The listing builds one solid part. Answer for the finished solid, in the listing's coordinates (mm). A direction names the side the tool comes from. Round coordinates to 2 decimals unless told otherwise and drop trailing zeros. Write each loop counter-clockwise with the first axis right and the second up, starting at its lowest first coordinate (ties: lowest second). Pieces come first, ordered by that corner, then holes.
(1) A cutting plane is placed at D-D, the plane y = 15. Give the vertices of the cut face in (x, z), and give its area (3 significant figures).
(2) Each of these flat-tipped pins is pushed along its axis until it touches: pin 1 Ø4 at (x, y) = (7, 7) entering from +Z; pin 2 Ø2 at (x, z) = (-1, 1) entering from -Y; pin 3 Ø2 at (y, z) = (11, 0) entering from +X. Where does it stop, or does it pass through?
(3) For faces 1 (the face through (-1, 1, 8)), 2 (the face through (-2.579, 4.93, -1.978)), 3 (the face through (-5, 0.49, -7.84)), determine the directions among +Z, -Z, +X, -X, +Y, -Y from which every point of the face is accessible in a straight line to the end or side of a thin tool.
(4) A cutting plane is placed at C-C, the plane z = 0. Give the vertices of the cut face in (x, y).
(5) Find the intervals of material crossed by probe 1 along Z at (x, y) = (0, 6.5); probe 2 along Y at (x, z) = (-2.75, -0.5); probe 3 along Y at (x, z) = (4.25, 6.5), in increasing order.
(6) The mould has two halves that part along Z. Classify faces 4 (the face through (0, 10, 0)), 5 (the face through (-4, 0, 0)), 6 (the face through (-7.493, 9.628, 0.33)): +Z half, -Z half, draft (parallel to the pull), parting line (faces both ways), or undercut.
(7) A cutting plane is placed at B-B, the plane x = 0. Give the vertices of the cut face in (y, z), and give its area (3 significant figures).
(8) A cutting plane is placed at A-A, the plane y = 8.25. Give the vertices of the cut face in (x, z).
Autodesk Inventor part; units mm, degrees
ref_plane "YZ Plane" through (0, 0, 0) normal (1, 0, 0) x (0, 1, 0)
ref_plane "XZ Plane" through (0, 0, 0) normal (0, 1, 0) x (-1, 0, 0)
ref_plane "XY Plane" through (0, 0, 0) normal (0, 0, 1) x (1, 0, 0)
sketch "Esboço1" plane through (0, 0, 0) normal (0, 1, 0) x (-1, 0, 0)
  circle A0 centre (0, 0) radius 9.3
  dimension "d0" = 18.6
extrude "Extrusão1" add sketch "Esboço1" along normal blind 1
sketch "Esboço2" plane through (0, 1, 0) normal (0, 1, 0) x (1, 0, 0)
  circle A0 centre (0, 0) radius 8.3
  circle A1 centre (0, 0) radius 9.3
  circle A2 centre (0, 0) radius 7.5
  dimension "d3" = 1
  dimension "d4" = 15
extrude "Extrusão2" add sketch "Esboço2" along normal blind 19.5 contours A2
fillet "Arredondamento1" radius 2 1 edges at (-7.5, 20.5, 0)
sketch "Esboço6" plane through (0, 0, 0) normal (0, -1, 0) x (1, 0, 0)
  circle A0 centre (0, 0) radius 3.25
  dimension "d13" = 6.5
extrude "Extrusão5" cut sketch "Esboço6" against normal blind 10
properties part number "Knob"
Solutions:
1. outline: circle Ø15 at (0, 0)
1. area: 177 mm2
2. pin 1: stops at z = 5.59
2. pin 2: stops at y = 10
2. pin 3: stops at x = 7.5
3. face 1: +Y
3. face 2: -Y
3. face 3: +Y, -Y
4. outline: (-9.3, 0) - (-3.25, 0) - (-3.25, 10) - (3.25, 10) - (3.25, 0) - (9.3, 0) - (9.3, 1) - (7.5, 1) - (7.5, 18.5) arc R2 ccw to (5.5, 20.5) - (-5.5, 20.5) arc R2 ccw to (-7.5, 18.5) - (-7.5, 1) - (-9.3, 1) - close
5. probe 1: z = -7.5 to -3.25, 3.25 to 7.5
5. probe 2: y = 10 to 20.5
5. probe 3: y = 0 to 1
6. face 4: undercut
6. face 5: draft
6. face 6: parting line
7. outline: (0, -9.3) - (1, -9.3) - (1, -7.5) - (18.5, -7.5) arc R2 ccw to (20.5, -5.5) - (20.5, 5.5) arc R2 ccw to (18.5, 7.5) - (1, 7.5) - (1, 9.3) - (0, 9.3) - (0, 3.25) - (10, 3.25) - (10, -3.25) - (0, -3.25) - close
7. area: 244 mm2
8. outline: circle Ø15 at (0, 0); hole circle Ø6.5 at (0, 0)
